from build123d import *

# Parameters (mm, degrees)
SKETCH_1_W          = 295
SKETCH_1_H          = 300
SKETCH_1_R          = 13
EXTRUDE_466_DEPTH   = 11.5
SKETCH_2_W          = 295
SKETCH_2_H          = 14
EXTRUDE_1_DEPTH     = 89
SKETCH_3_R          = 13
CUT_EXTRUDE_1_DEPTH = 346.943998358


with BuildPart() as part:
    # 草图1 → Extrude 466 (new body)
    with BuildSketch(Plane.XY):
        with Locations((0, 150)):
            Rectangle(SKETCH_1_W, SKETCH_1_H)
        with Locations((92.5, 230)):
            Circle(SKETCH_1_R, mode=Mode.SUBTRACT)
        with Locations((92.5, 150)):
            Circle(SKETCH_1_R, mode=Mode.SUBTRACT)
        with Locations((92.5, 70)):
            Circle(SKETCH_1_R, mode=Mode.SUBTRACT)
        with Locations((12.5, 230)):
            Circle(SKETCH_1_R, mode=Mode.SUBTRACT)
        with Locations((-67.5, 230)):
            Circle(SKETCH_1_R, mode=Mode.SUBTRACT)
        with Locations((-67.5, 150)):
            Circle(SKETCH_1_R, mode=Mode.SUBTRACT)
        with Locations((-67.5, 70)):
            Circle(SKETCH_1_R, mode=Mode.SUBTRACT)
        with Locations((12.5, 70)):
            Circle(SKETCH_1_R, mode=Mode.SUBTRACT)
        with Locations((12.5, 150)):
            Circle(SKETCH_1_R, mode=Mode.SUBTRACT)
    extrude(amount=EXTRUDE_466_DEPTH)

    # 草图2 → 凸台-拉伸1 (add)
    with BuildSketch(Plane(origin=(0, 0, 0), x_dir=(-1, 0, 0), z_dir=(0, 0, -1))):
        with Locations((0, 293)):
            Rectangle(SKETCH_2_W, SKETCH_2_H)
        with Locations((0, 7)):
            Rectangle(SKETCH_2_W, SKETCH_2_H)
    extrude(amount=EXTRUDE_1_DEPTH)

    # 草图3 → 切除-拉伸1 (cut, through all)
    with BuildSketch(Plane(origin=(0, 300, 0), x_dir=(-1, 0, 0), z_dir=(0, 1, 0))):
        with Locations(Location((-27.5, -53.5, 0), (0, 0, 90))):
            Circle(SKETCH_3_R)
        with Locations(Location((52.5, -53.5, 0), (0, 0, 90))):
            Circle(SKETCH_3_R)
    extrude(amount=-CUT_EXTRUDE_1_DEPTH, mode=Mode.SUBTRACT)


solid = part.part
Input: part model. Units: mm. Frame: model coordinates. A direction names the side the tool comes from. Round coordinates to 2 decimals unless told otherwise and drop trailing zeros. Write each loop counter-clockwise with the first axis right and the second up, starting at its lowest first coordinate (ties: lowest second). Pieces come first, ordered by that corner, then holes.
1) Cut plane B-B (z = -74). Return the cut outline in (x, y), then the cut area to 3 significant figures.
2) Cut plane A-A (z = -53.5). Return the cut outline in (x, y), then the cut area to 3 significant figures.
3) Ray query, L1, parallel to Y at x = 12.5, z = 8.25; L2, parallel to Y at x = 68, z = -2.5; L3, parallel to X at y = 292.5, z = -53.5. Return the intervals inside material, ascending.
4) Reachability of faces 4 (the flat face through (-2, 152, 11.5)), 5 (the flat face through (-2, 152, 0)) from +Z, -Z, +X, -X, +Y, -Y: full face, straight path, thin tool, end or side. Return the list, or none.
5) Cut plane D-D (x = -10.5). Return the cut outline in (y, z).
6) Contact query for a flat-ended pin moving along its axis: P1, Ø3, axis at x = -90, y = 69, coming from the -Z side. Output: stop coordinate, or through.
7) Draft query along X for faces 1 (the flat face through (147.5, 149, 2)), 2 (the flat face through (2, 7, -89)), 3 (the cylindrical face through (10.81, 242.89, 5.67)). Return one class per face: pulls with the +X half, pulls with the -X half, needs draft (parallel to the pull), parting line crosses it, or undercut.
8) Cut plane C-C (y = 70). Return the cut outline in (x, z).
Geometry says:
1. outline: (-147.5, 0) - (147.5, 0) - (147.5, 14) - (-147.5, 14) - close; (-147.5, 286) - (147.5, 286) - (147.5, 300) - (-147.5, 300) - close
1. area: 8,260 mm2
2. outline: (-147.5, 0) - (-65.5, 0) - (-65.5, 14) - (-147.5, 14) - close; (-147.5, 286) - (-65.5, 286) - (-65.5, 300) - (-147.5, 300) - close; (-39.5, 0) - (14.5, 0) - (14.5, 14) - (-39.5, 14) - close; (-39.5, 286) - (14.5, 286) - (14.5, 300) - (-39.5, 300) - close; (40.5, 0) - (147.5, 0) - (147.5, 14) - (40.5, 14) - close; (40.5, 286) - (147.5, 286) - (147.5, 300) - (40.5, 300) - close
2. area: 6,800 mm2
3. L1: y = 0 to 57, 83 to 137, 163 to 217, 243 to 300
3. L2: y = 0 to 14, 286 to 300
3. L3: x = -147.5 to -65.5, -39.5 to 14.5, 40.5 to 147.5
4. face 4: +Z, +X, -X, +Y, -Y
4. face 5: -Z, +X, -X
5. outline: (0, -89) - (14, -89) - (14, 0) - (286, 0) - (286, -89) - (300, -89) - (300, 11.5) - (0, 11.5) - close
6. P1: stops at z = 0
7. face 1: pulls with the +X half
7. face 2: needs draft
7. face 3: undercut
8. outline: (-147.5, 0) - (-80.5, 0) - (-80.5, 11.5) - (-147.5, 11.5) - close; (-54.5, 0) - (-0.5, 0) - (-0.5, 11.5) - (-54.5, 11.5) - close; (25.5, 0) - (79.5, 0) - (79.5, 11.5) - (25.5, 11.5) - close; (105.5, 0) - (147.5, 0) - (147.5, 11.5) - (105.5, 11.5) - close
